Verification items for the finished model (mm, model axes). A direction names the side the tool comes from. Round coordinates to 2 decimals unless told otherwise and drop trailing zeros. Loops run counter-clockwise (first coordinate to the right, second up) from the corner with the lowest first, then second, coordinate; pieces in that order, holes last. Notation, with made-up numbers: (66.25, -1.5) -> (72.25, -1.5) arc R17 ccw to (72.25, 8.5) -> close; hole circle Ø1 at (-22.5, -8.5). An arc over 180 degrees is marked (long way). Use a Markdown table: item, result. Add a question column.
```python
from build123d import *

# Parameters (mm, degrees)
SKETCH1_W           = 80
SKETCH1_H           = 30
BOSS_EXTRUDE1_DEPTH = 50
SKETCH2_W           = 50
SKETCH2_H           = 20
CUT_EXTRUDE1_DEPTH  = 50
SKETCH3_R           = 2.5
CUT_EXTRUDE2_DEPTH  = 50


with BuildPart() as part:
    # Sketch1 → Boss-Extrude1 (new body)
    with BuildSketch(Plane.XY):
        Rectangle(SKETCH1_W, SKETCH1_H)
    extrude(amount=BOSS_EXTRUDE1_DEPTH)

    # Sketch2 → Cut-Extrude1 (cut)
    with BuildSketch(Plane.XY.offset(50)):
        with Locations((0, -5)):
            Rectangle(SKETCH2_W, SKETCH2_H)
    extrude(amount=-CUT_EXTRUDE1_DEPTH, mode=Mode.SUBTRACT)

    # Sketch3 → Cut-Extrude2 (cut)
    with BuildSketch(Plane.XY.offset(50)):
        with Locations((-32.5, 0)):
            Circle(SKETCH3_R)
        with Locations((32.5, 0)):
            Circle(SKETCH3_R)
    extrude(amount=-CUT_EXTRUDE2_DEPTH, mode=Mode.SUBTRACT)


solid = part.part
```
1) Sectioned sample at C-C on x = -32.5. Enter the section's corners in (y, z), then the cut area to 3 significant figures.
2) Sectioned sample at B-B on y = -4.25. Enter the section's corners in (x, z), then the cut area to 3 significant figures.
3) Go/stop test with a flat-tipped pin: pin 1 (15 mm diameter, centred on x = 7.5, z = 17.5, fed in from -Y). Record where the tip stops, or that it passes through.
4) Release check for a two-part mould opening along X. For faces 1 (the face through (25, -5, 25)), 2 (the face through (40, 0, 25)), 3 (the face through (-35, 0, 25)), 4 (the face through (-1, 15, 25)) record: released by +X, released by -X, zero draft, split by the parting line, or undercut.
5) Sectioned sample at D-D on y = 0. Enter the section's corners in (x, z).
6) Sectioned sample at A-A on z = 29. Enter the section's corners in (x, y), then the cut area to 3 significant figures.
7) Thickness scan on line 1 (X direction, y = 3.5, z = 5.5); line 2 (X direction, y = 0.5, z = 16); line 3 (Y direction, x = 32.5, z = 27). Record the ranges inside material, lowest first.
8) Access from +Z, -Z, +X, -X, +Y, -Y to the whole of each face (thin tool, end or side, straight path). Record for faces 5 (the face through (-1, 7, 0)), 6 (the face through (0, 5, 25)).
Geometry results:
| question | item | result |
|---|---|---|
| 1 | outline | (-15, 0) -> (-2.5, 0) -> (-2.5, 50) -> (-15, 50) -> close; (2.5, 0) -> (15, 0) -> (15, 50) -> (2.5, 50) -> close |
| 1 | area | 1,250 mm^2 |
| 2 | outline | (-40, 0) -> (-25, 0) -> (-25, 50) -> (-40, 50) -> close; (25, 0) -> (40, 0) -> (40, 50) -> (25, 50) -> close |
| 2 | area | 1,500 mm^2 |
| 3 | pin 1 | y = 5 |
| 4 | face 1 | undercut |
| 4 | face 2 | released by +X |
| 4 | face 3 | undercut |
| 4 | face 4 | zero draft |
| 5 | outline | (-40, 0) -> (-35, 0) -> (-35, 50) -> (-40, 50) -> close; (-30, 0) -> (-25, 0) -> (-25, 50) -> (-30, 50) -> close; (25, 0) -> (30, 0) -> (30, 50) -> (25, 50) -> close; (35, 0) -> (40, 0) -> (40, 50) -> (35, 50) -> close |
| 6 | outline | (-40, -15) -> (-25, -15) -> (-25, 5) -> (25, 5) -> (25, -15) -> (40, -15) -> (40, 15) -> (-40, 15) -> close; hole circle Ø5 at (-32.5, 0); hole circle Ø5 at (32.5, 0) |
| 6 | area | 1,360 mm^2 |
| 7 | line 1 | -40 to -25, 25 to 40 |
| 7 | line 2 | -40 to -34.95, -30.05 to -25, 25 to 30.05, 34.95 to 40 |
| 7 | line 3 | -15 to -2.5, 2.5 to 15 |
| 8 | face 5 | -Z, +X, -X, +Y, -Y |
| 8 | face 6 | +Z, -Z, -Y |
